Source: CAD feature listing. Evaluate the final solid. Frame: model axes, mm. Face numbers are marked on the shaded views. A direction names the side the tool comes from. Give positions to 0.01 mm unless a question says otherwise; leave off trailing zeros. Order: outer loops, then holes, each group sorted by start corner. A loop starts at its lowest first (then second) coordinate and runs counter-clockwise, first axis right, second up. Notation, with made-up numbers: M 54.25,-14 L 84.25,-14 A17 ccw 84.25,12 Z; hole C 78,-36.75 d9. An arc over 180 degrees is marked long. Return JSON: item names as keys, results as strings.
Autodesk Inventor part; units mm, degrees
ref_plane "Work Plane1" through (0, 0, 60) normal (0, 0, 1) x (1, 0, 0)
ref_plane "YZ Plane" through (0, 0, 0) normal (1, 0, 0) x (0, 1, 0)
ref_plane "XZ Plane" through (0, 0, 0) normal (0, 1, 0) x (-1, 0, 0)
sketch "Sketch1" plane through (0, 0, 0) normal (0, 0, 1) x (1, 0, 0)
  line L0 (-37.2, 47) -> (37.2, 47)
  line L1 (47, 37.2) -> (47, -37.2)
  line L2 (37.2, -47) -> (-37.2, -47)
  line L3 (-47, -37.2) -> (-47, 37.2)
  circle A0 centre (0, 0) radius 52.5 construction
  line L4 (-37.125, 58) -> (-37.125, -64) construction
  line L5 (37.125, 58) -> (37.125, -64) construction
  line L6 (-69, 37.125) -> (85, 37.125) construction
  line L7 (-58, -37.125) -> (77, -37.125) construction
  circle A1 centre (-37.125, 37.125) radius 3.175
  circle A2 centre (37.125, 37.125) radius 3.175
  circle A3 centre (37.125, -37.125) radius 3.175
  circle A4 centre (-37.125, -37.125) radius 3.175
  line L8 (-37.2, 47) -> (-47, 37.2)
  line L9 (37.2, 47) -> (47, 37.2)
  line L10 (-47, -37.2) -> (-37.2, -47)
  line L11 (37.2, -47) -> (47, -37.2)
  point P0 (-47, 47)
  point P1 (47, -47)
  point P2 (47, 47)
  point P3 (-47, -47)
  dimension "d0" = 94
  dimension "d1" = 47
  dimension "d2" = 47
  dimension "d3" = 105
  dimension "d4" = 74.25
  dimension "d5" = 37.125
  dimension "d6" = 74.25
  dimension "d7" = 37.125
  dimension "d8" = 6.35
  dimension "d9" = 6.35
  dimension "d10" = 6.35
  dimension "d11" = 6.35
  dimension "d12" = 9.8
  dimension "d13" = 9.8
  dimension "d14" = 9.8
  dimension "d15" = 9.8
  dimension "d16" = 9.8
  dimension "d17" = 9.8
  dimension "d18" = 9.8
  dimension "d19" = 9.8
extrude "Extrusion1" add sketch "Sketch1" along normal blind 10
sketch "Sketch2" plane through (0, 0, 10) normal (0, 0, 1) x (1, 0, 0)
  circle A0 centre (0, 0) radius 40
  dimension "d22" = 80
extrude "Extrusion2" add sketch "Sketch2" along normal blind 5
sketch "Sketch3" plane through (0, 0, 15) normal (0, 0, 1) x (1, 0, 0)
  circle A0 centre (0, 0) radius 10
  dimension "d25" = 20
extrude "Extrusion3" add sketch "Sketch3" along normal blind 50
ref_plane "Work Plane1" through (0, 0, 60) normal (0, 0, 1) x (1, 0, 0)
sketch "Sketch5" plane through (0, 0, 60) normal (0, 0, 1) x (1, 0, 0)
  line L0 (-3, 12.5) -> (3, 12.5)
  line L1 (3, 12.5) -> (3, 7.2)
  line L2 (3, 7.2) -> (-3, 7.2)
  line L3 (-3, 7.2) -> (-3, 12.5)
  point P0 (0, 0)
  dimension "d29" = 6
  dimension "d30" = 3
  dimension "d31" = 12.5
extrude "Extrusion4" add sketch "Sketch5" against normal blind 25
sketch "Sketch6" plane through (0, 0, 0) normal (0, 0, -1) x (-1, 0, 0)
  circle A0 centre (0, 0) radius 45
  dimension "d34" = 90
extrude "Extrusion5" add sketch "Sketch6" along normal blind 51
sketch "Sketch8" plane through (0, 0, -51) normal (0, 0, -1) x (-1, 0, 0)
  line L0 (-37.2, 47) -> (37.2, 47)
  line L1 (47, 37.2) -> (47, -37.2)
  line L2 (37.2, -47) -> (-37.2, -47)
  line L3 (-47, -37.2) -> (-47, 37.2)
  line L4 (-37.2, 47) -> (37.2, 47)
  line L5 (47, 37.2) -> (47, -37.2)
  line L6 (37.2, -47) -> (-37.2, -47)
  line L7 (-47, -37.2) -> (-47, 37.2)
  circle A0 centre (-34.798, 34.798) radius 2.5
  circle A1 centre (34.798, 34.798) radius 2.5
  circle A2 centre (34.798, -34.798) radius 2.5
  circle A3 centre (-34.798, -34.798) radius 2.5
  line L8 (-37.2, 47) -> (-47, 37.2)
  line L9 (37.2, 47) -> (47, 37.2)
  line L10 (47, -37.2) -> (37.2, -47)
  line L11 (-37.2, -47) -> (-47, -37.2)
  point P0 (0, 0)
  point P1 (-47, 47)
  point P2 (47, -47)
  point P3 (47, 47)
  point P4 (-47, -47)
  dimension "d38" = 5
  dimension "d39" = 5
  dimension "d40" = 5
  dimension "d41" = 5
  dimension "d42" = 69.596
  dimension "d43" = 69.596
  dimension "d44" = 69.596
  dimension "d45" = 69.596
  dimension "d46" = 34.798
  dimension "d47" = 34.798
  dimension "d48" = 34.798
  dimension "d49" = 34.798
  dimension "d50" = 9.8
  dimension "d51" = 9.8
  dimension "d52" = 9.8
  dimension "d53" = 9.8
  dimension "d54" = 9.8
  dimension "d55" = 9.8
  dimension "d56" = 9.8
  dimension "d57" = 9.8
extrude "Extrusion6" add sketch "Sketch8" along normal blind 56
sketch "Sketch9" plane through (0, 0, -107) normal (0, 0, -1) x (-1, 0, 0)
  circle A0 centre (0, 0) radius 6.35
  dimension "d60" = 12.7
extrude "Extrusion7" cut sketch "Sketch9" against normal blind 40
properties part number "1224a_Stepper Motor Gearbox_V1"
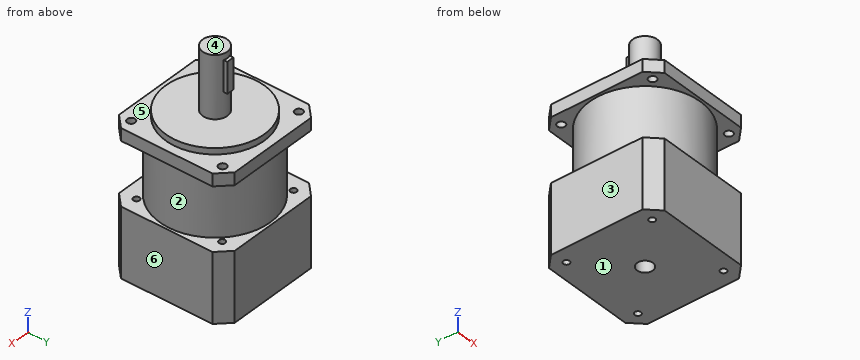
1. Section query C-C (z = -15.5). Return loops of the section in (x, y).
Evaluation:
{"outline": "C 0,0 d90"}
2. Draft query along Z for the marked faces 1, 2, 3 and 4. Return one class per face: pulls with the +Z half, pulls with the -Z half, needs draft (parallel to the pull), parting line crosses it, or undercut.
Evaluation:
{"face 1": "pulls with the -Z half", "face 2": "undercut", "face 3": "needs draft", "face 4": "pulls with the +Z half"}
3. First-contact query: pin 1 (3.5 mm diameter, centred on y = 11, z = 48, fed in from -X); pin 2 (2 mm diameter, centred on x = -20, y = -33, fed in from +Z); pin 3 (4.5 mm diameter, centred on x = -34.798, y = 34.798, fed in from -Z). Flat tips, straight axial feed; report the tip coordinate or a pass-through.
Evaluation:
{"pin 1": "stops at x = -3.8", "pin 2": "stops at z = 15", "pin 3": "stops at z = 0"}
4. Ray query, probe 1 along Y at (x, z) = (0.5, -87); probe 2 along Z at (x, y) = (-43, 18); probe 3 along Z at (x, y) = (-5.5, 31.5). Return the intervals inside material, ascending.
Evaluation:
{"probe 1": "y = -47 to -6.33, 6.33 to 47", "probe 2": "z = -107 to -51, 0 to 10", "probe 3": "z = -107 to 15"}
5. Section query D-D (x = 18.5). Return loops of the section in (y, z), then the cut area to 3 significant figures.
Evaluation:
{"outline": "M -47,-107 L 47,-107 L 47,-51 L 41.02,-51 L 41.02,0 L 47,0 L 47,10 L 35.46,10 L 35.46,15 L -35.46,15 L -35.46,10 L -47,10 L -47,0 L -41.02,0 L -41.02,-51 L -47,-51 Z", "area": "10,700 mm^2"}
6. Section query A-A (x = 0). Return loops of the section in (y, z).
Evaluation:
{"outline": "M -47,-107 L -6.35,-107 L -6.35,-67 L 6.35,-67 L 6.35,-107 L 47,-107 L 47,-51 L 45,-51 L 45,0 L 47,0 L 47,10 L 40,10 L 40,15 L 10,15 L 10,35 L 12.5,35 L 12.5,60 L 10,60 L 10,65 L -10,65 L -10,15 L -40,15 L -40,10 L -47,10 L -47,0 L -45,0 L -45,-51 L -47,-51 Z"}
7. Section query B-B (y = 0). Return loops of the section in (x, z).
Evaluation:
{"outline": "M -47,-107 L -6.35,-107 L -6.35,-67 L 6.35,-67 L 6.35,-107 L 47,-107 L 47,-51 L 45,-51 L 45,0 L 47,0 L 47,10 L 40,10 L 40,15 L 10,15 L 10,65 L -10,65 L -10,15 L -40,15 L -40,10 L -47,10 L -47,0 L -45,0 L -45,-51 L -47,-51 Z"}
8. Set-up query: the marked faces 5 and 6. Return all of +Z, -Z, +X, -X, +Y, -Y with unobstructed straight access to the full face (end or side cutting, diameter ignored); none if empty.
Evaluation:
{"face 5": "+Z", "face 6": "+Z, -Z, +X, +Y, -Y"}
